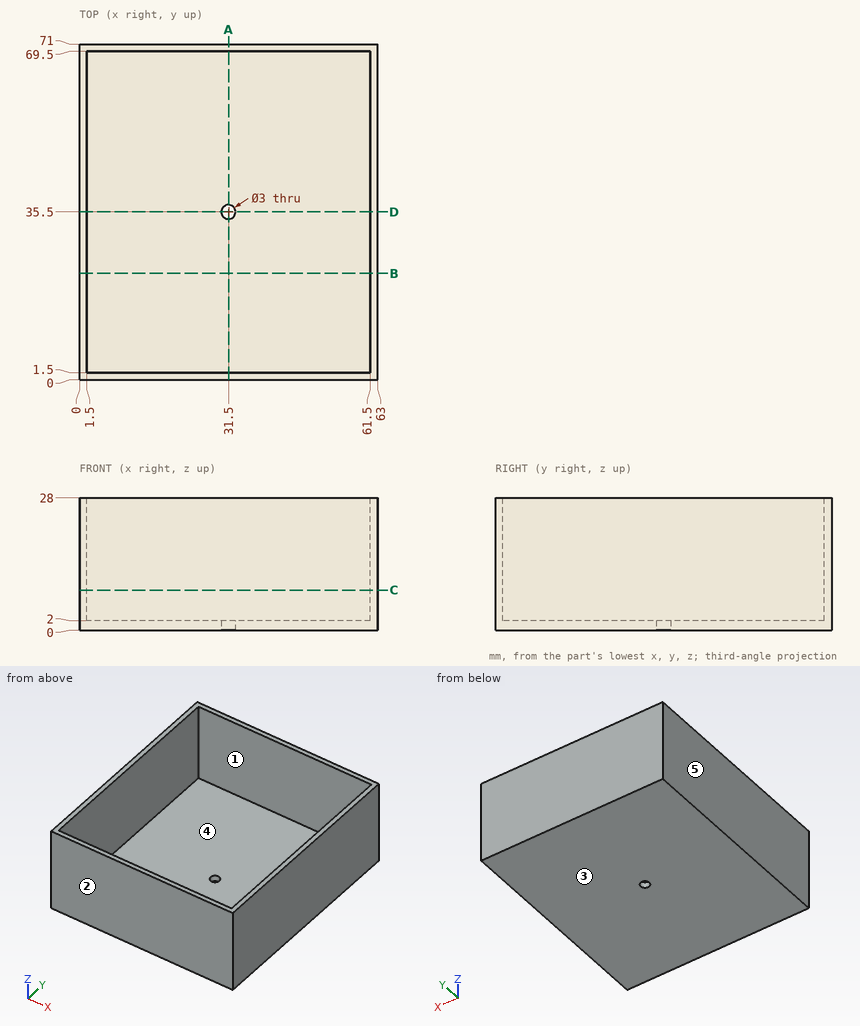
Answer from the drawing. Dimensions are ordinates in mm from the lowest x, y and z of the part. A direction names the side the tool comes from. Give positions to 0.01 mm unless a question says otherwise; leave off trailing zeros. Write each loop counter-clockwise with the first axis right and the second up, starting at its lowest first coordinate (ties: lowest second). Pieces come first, ordered by that corner, then holes. Notation, with made-up numbers: (18.25, 23.25) - (24.25, 23.25) arc R15 cw to (24.25, 35.25) - close; hole circle Ø1 at (71, 67). An arc over 180 degrees is marked (long way). One line per item, written item: value. Start each with the question number.
1. For a pull along Y with two mould halves and no side action, classify the marked faces 1, 2 and 3 as +Y half, -Y half, draft (parallel to the pull), parting line (faces both ways), or undercut.
2. Find section D-D (y = 35.5). Write down the section's boundary in (x, z).
3. Consider probe 1 along Y at (x, z) = (44, 21.5); probe 2 along X at (y, z) = (51, 14); probe 3 along Y at (x, z) = (31.5, 1.5). Determine where each line is inside the solid, lowest interval first.
4. Find section A-A (x = 31.5). Write down the section's boundary in (y, z), then the cut area to 3 significant figures.
5. For the marked faces 4 and 5, determine the directions among +Z, -Z, +X, -X, +Y, -Y from which every point of the face is accessible in a straight line to the end or side of a thin tool.
6. Find section C-C (z = 8.5). Write down the section's boundary in (x, y), then the cut area to 3 significant figures.
7. Find section B-B (y = 22.5). Write down the section's boundary in (x, z).
8. Given pin 1 (4 mm diameter, centred on x = 28, y = 13.5, fed in from +Z), flat-ended and moving along its own axis, determine where the tip first touches the part or whether it passes through.
Geometry results:
1. face 1: undercut
1. face 2: -Y half
1. face 3: draft
2. outline: (0, 0) - (30, 0) - (30, 2) - (1.5, 2) - (1.5, 28) - (0, 28) - close; (33, 0) - (63, 0) - (63, 28) - (61.5, 28) - (61.5, 2) - (33, 2) - close
3. probe 1: 0 to 1.5, 69.5 to 71
3. probe 2: 0 to 1.5, 61.5 to 63
3. probe 3: 0 to 34, 37 to 71
4. outline: (0, 0) - (34, 0) - (34, 2) - (1.5, 2) - (1.5, 28) - (0, 28) - close; (37, 0) - (71, 0) - (71, 28) - (69.5, 28) - (69.5, 2) - (37, 2) - close
4. area: 214 mm2
5. face 4: +Z
5. face 5: +Z, -Z, -X, +Y, -Y
6. outline: (0, 0) - (63, 0) - (63, 71) - (0, 71) - close; hole (1.5, 1.5) - (61.5, 1.5) - (61.5, 69.5) - (1.5, 69.5) - close
6. area: 393 mm2
7. outline: (0, 0) - (63, 0) - (63, 28) - (61.5, 28) - (61.5, 2) - (1.5, 2) - (1.5, 28) - (0, 28) - close
8. pin 1: z = 2
